from build123d import *

# Parameters (mm, degrees)
SKETCH1_W           = 3
SKETCH1_H           = 8
BOSS_EXTRUDE1_DEPTH = 3
SKETCH2_W           = 4
SKETCH2_H           = 3
BOSS_EXTRUDE2_DEPTH = 4
SKETCH4_W           = 7
SKETCH4_H           = 4
BOSS_EXTRUDE3_DEPTH = 2
CUT_EXTRUDE2_REACH  = 10.441
SKETCH5_R           = 0.75
FILLET4_R           = 1.5


with BuildPart() as part:
    # Sketch1 → Boss-Extrude1 (new body)
    with BuildSketch(Plane(origin=(0, 0, 0), x_dir=(1, 0, 0), z_dir=(0, 1, 0))):
        Rectangle(SKETCH1_W, SKETCH1_H)
    extrude(amount=BOSS_EXTRUDE1_DEPTH)

    # Sketch2 → Boss-Extrude2 (add)
    with BuildSketch(Plane(origin=(1.5, 0, 0), x_dir=(0, 0, -1), z_dir=(1, 0, 0))):
        with Locations((-2, 1.5)):
            Rectangle(SKETCH2_W, SKETCH2_H)
    extrude(amount=BOSS_EXTRUDE2_DEPTH)

    # Sketch4 → Boss-Extrude3 (add)
    with BuildSketch(Plane(origin=(0, 3, 0), x_dir=(-1, 0, 0), z_dir=(0, -1, 0))):
        with Locations((-2, -2)):
            Rectangle(SKETCH4_W, SKETCH4_H)
    extrude(amount=-BOSS_EXTRUDE3_DEPTH)

    # Sketch5 → Cut-Extrude2 (cut, up to next)
    with BuildSketch(Plane(origin=(0, 5, 0), x_dir=(1, 0, 0), z_dir=(0, 1, 0)), mode=Mode.PRIVATE) as cut_extrude2_sk1:
        with Locations(Location((0, -2, 0), (0, 0, 270))):
            Circle(SKETCH5_R)
    cut_extrude2_tool1 = extrude(cut_extrude2_sk1.sketch, amount=-CUT_EXTRUDE2_REACH, mode=Mode.PRIVATE) & part.part
    # Sketch5 → Cut-Extrude2 (cut, up to next)
    with BuildSketch(Plane(origin=(0, 5, 0), x_dir=(1, 0, 0), z_dir=(0, 1, 0)), mode=Mode.PRIVATE) as cut_extrude2_sk2:
        with Locations(Location((4, -2, 0), (0, 0, 270))):
            Circle(SKETCH5_R)
    cut_extrude2_tool2 = extrude(cut_extrude2_sk2.sketch, amount=-CUT_EXTRUDE2_REACH, mode=Mode.PRIVATE) & part.part
    add(cut_extrude2_tool1.solids().sort_by_distance((0, 5, 2))[0], mode=Mode.SUBTRACT)
    add(cut_extrude2_tool2.solids().sort_by_distance((4, 5, 2))[0], mode=Mode.SUBTRACT)

    # Fillet4
    # the kernel refuses this fillet: 1.5 mm, written as the material it takes off along each edge
    with BuildSketch(Plane(origin=(1.5, 0, -7.75), x_dir=(-1, 0, 0), z_dir=(0, 0, 1)), Plane(origin=(1.5, 3, -7.75), x_dir=(0, -1, 0), z_dir=(0, 0, 1)), Plane(origin=(-1.5, 3, 0), x_dir=(0, -1, 0), z_dir=(0, 0, -1))) as fillet4_piece_1:
        with BuildLine():
            CenterArc((FILLET4_R, -FILLET4_R), FILLET4_R, 90, 90)
            Line((0, -FILLET4_R), (0, 0))
            Line((0, 0), (FILLET4_R, 0))
        make_face()
    extrude(amount=7.75, mode=Mode.SUBTRACT)
    with BuildSketch(Plane(origin=(-1.5, 0, 7.75), x_dir=(1, 0, 0), z_dir=(0, 0, -1))) as fillet4_piece_2:
        with BuildLine():
            CenterArc((FILLET4_R, -FILLET4_R), FILLET4_R, 90, 90)
            Line((0, -FILLET4_R), (0, 0))
            Line((0, 0), (FILLET4_R, 0))
        make_face()
    extrude(amount=15.5, mode=Mode.SUBTRACT)


solid = part.part
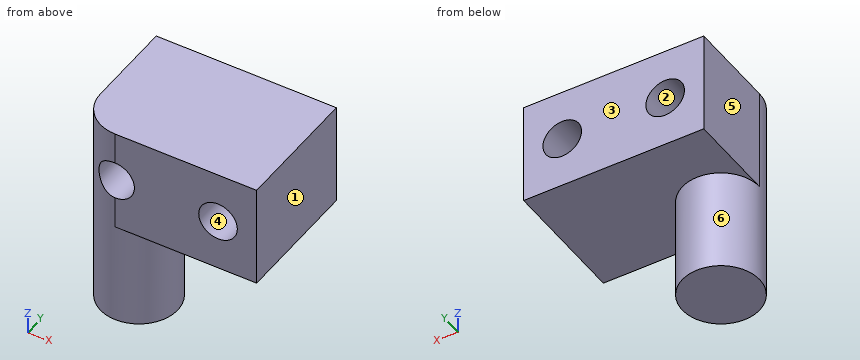
The model under review builds one solid part; all positions refer to its coordinate system, in mm. Face numbers are marked on the shaded views. A direction names the side the tool comes from. Round coordinates to 2 decimals unless told otherwise and drop trailing zeros. Loops run counter-clockwise (first coordinate to the right, second up) from the corner with the lowest first, then second, coordinate; pieces in that order, holes last. Notation, with made-up numbers: (62.5, 10) - (85.5, 10) arc R17 cw to (85.5, 30) - close; hole circle Ø7 at (-22, -13.5). An arc over 180 degrees is marked (long way). Use CSV: the item, a comma, the result in double quotes.
(1) Take a section at A-A, the plane x = 4. Give the boundary of the cut face in (y, z).
Working result:
outline,"(0, 0) - (5, 0) - (5, 1.25) - (0, 1.25) - close; (0, 2.75) - (5, 2.75) - (5, 4) - (0, 4) - close"
(2) The part is to be moulded in two halves that separate along X. For the marked faces 1, 2, 3 and 4, say which applies: pulls with the +X half, pulls with the -X half, needs draft (parallel to the pull), parting line crosses it, or undercut.
Working result:
face 1,"pulls with the +X half"
face 2,"undercut"
face 3,"needs draft"
face 4,"undercut"
(3) Machinability: for the marked faces 5 and 6, which of the approach directions +Z, -Z, +X, -X, +Y, -Y give a long, thin tool a straight path to every point of the face, cutting with its end or side? Answer none if there is none.
Working result:
face 5,"+Z, -Z, -X, +Y, -Y"
face 6,"-Z"
(4) For line 1 (X direction, y = 3.2, z = 2); line 2 (X direction, y = 4.3, z = 1.5); line 3 (Z direction, x = 0, y = 1.3), list the stretches that pass through material, from the lowest coordinate up.
Working result:
line 1,"x = -1.5 to -0.75, 0.75 to 3.25, 4.75 to 5.5"
line 2,"x = -1.5 to -0.56, 0.56 to 3.44, 4.56 to 5.5"
line 3,"z = -4 to 1.25, 2.75 to 4"
(5) Take a section at B-B, the plane z = 2. Give the boundary of the cut face in (x, y).
Working result:
outline,"(-1.5, 1.5) arc R1.5 ccw to (-0.75, 0.2) - (-0.75, 5) - (-1.5, 5) - close; (0.75, 0) - (3.25, 0) - (3.25, 5) - (0.75, 5) - close; (4.75, 0) - (5.5, 0) - (5.5, 5) - (4.75, 5) - close"
(6) Take a section at C-C, the plane y = 4.55. Give the boundary of the cut face in (x, z), plus the area to 3 significant figures.
Working result:
outline,"(-1.5, 0) - (5.5, 0) - (5.5, 4) - (-1.5, 4) - close; hole circle Ø1.5 at (0, 2); hole circle Ø1.5 at (4, 2)"
area,"24.5 mm^2"
(7) Take a section at D-D, the plane x = -0.25. Give the boundary of the cut face in (y, z), plus the area to 3 significant figures.
Working result:
outline,"(0.02, -4) - (2.98, -4) - (2.98, 0) - (5, 0) - (5, 1.29) - (0.02, 1.29) - close; (0.02, 2.71) - (5, 2.71) - (5, 4) - (0.02, 4) - close"
area,"24.7 mm^2"
(8) Clearance check with flat-ended pins moving along their axes: P1, Ø0.9, axis at x = 0, z = 2, coming from the -Y side; P2, Ø2, axis at x = 1.5, z = -2, coming from the +Y side. State where each tip first meets the part, or that it passes through.
Working result:
P1,"passes through"
P2,"stops at y = 2.91"
